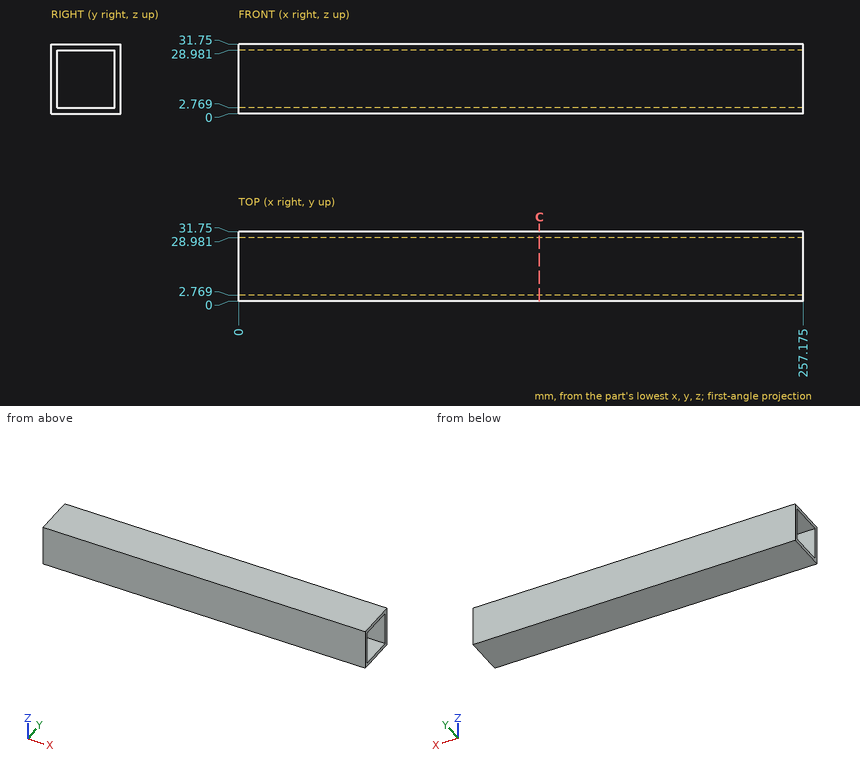
Check sheet for the drawn part. Datum: minimum x, y, z corner. Units: mm. Coordinates: 2 decimals unless noted, no trailing zeros. Loops run counter-clockwise (first coordinate to the right, second up) from the corner with the lowest first, then second, coordinate; pieces in that order, holes last. Notation, with made-up numbers: (84.25, 5.5) -> (97.25, 5.5) arc R32 ccw to (97.25, 39.5) -> close; hole circle Ø8 at (76.5, 70.5). An arc over 180 degrees is marked (long way). Answer in a Markdown table with one row per item.
1. Material ranges on line 1 along Y through (x, z) = (67, 21), recorded low to high. Write a range as [from, to].
Check values:
| item | result |
|---|---|
| line 1 | y = [0, 2.77], [28.98, 31.75] |
2. Sectioned sample at C-C, the plane x = 137. Record the boundary of the cut face in (y, z).
Check values:
| item | result |
|---|---|
| outline | (0, 0) -> (31.75, 0) -> (31.75, 31.75) -> (0, 31.75) -> close; hole (2.77, 2.77) -> (28.98, 2.77) -> (28.98, 28.98) -> (2.77, 28.98) -> close |
3. Go/stop test with flat-tipped pins: pin 1 (6 mm diameter, centred on y = 25.5, z = 10.5, fed in from +X); pin 2 (13 mm diameter, centred on x = 76, y = 13, fed in from -Z). Record where each tip stops, or that it passes through.
Check values:
| item | result |
|---|---|
| pin 1 | passes through |
| pin 2 | stops at z = 0 |
